```python
from build123d import *

# Parameters (mm, degrees)
SKETCH1_W           = 40
SKETCH1_H           = 40
BOSS_EXTRUDE1_DEPTH = 20
CUT_EXTRUDE1_START  = 13
SKETCH2_R           = 2.05
CUT_EXTRUDE1_DEPTH  = 34
BOSS_EXTRUDE2_DEPTH = 10
FILLET1_R           = 10
CHAMFER1_SIZE       = 1
FILLET2_R           = 3


with BuildPart() as part:
    # Sketch1 → Boss-Extrude1 (new body, symmetric)
    with BuildSketch(Plane(origin=(0, 0, 0), x_dir=(1, 0, 0), z_dir=(0, 1, 0))):
        Rectangle(SKETCH1_W, SKETCH1_H)
    extrude(amount=BOSS_EXTRUDE1_DEPTH, both=True)

    # Sketch2 → Cut-Extrude1 (cut, through all)
    with BuildSketch(Plane(origin=(0, 0, 0), x_dir=(0, 0, -1), z_dir=(1, 0, 0)).offset(CUT_EXTRUDE1_START)):
        with Locations((-7.5, 10)):
            Circle(SKETCH2_R)
        with Locations((7.5, 10)):
            Circle(SKETCH2_R)
        with Locations((-7.5, -10)):
            Circle(SKETCH2_R)
        with Locations((7.5, -10)):
            Circle(SKETCH2_R)
    cut_extrude1 = extrude(amount=-CUT_EXTRUDE1_DEPTH, mode=Mode.SUBTRACT)

    # Mirror1: Cut-Extrude1 across plane
    add(cut_extrude1.mirror(Plane(origin=(0, 0, 0), x_dir=(0, 0, 1), z_dir=(1, 0, 0))), mode=Mode.SUBTRACT)

    # Sketch3 → Boss-Extrude2 (add)
    with BuildSketch(Plane(origin=(0, 20, 0), x_dir=(1, 0, 0), z_dir=(0, 1, 0))):
        with BuildLine():
            Line((18.68, 3.6), (8.4, 3.6))
            Line((8.4, 3.6), (8.4, -3.6))
            Line((8.4, -3.6), (18.68, -3.6))
            ThreePointArc((18.68, -3.6), (19.408599647, -3.761942699), (20, -4.2172761))
            Line((20, -4.2172761), (20, 4.2172761))
            ThreePointArc((20, 4.2172761), (19.408599647, 3.761942699), (18.68, 3.6))
        make_face()
        with BuildLine():
            ThreePointArc((3.6, 18.68), (3.761942699, 19.408599647), (4.2172761, 20))
            Line((4.2172761, 20), (-4.2172761, 20))
            ThreePointArc((-4.2172761, 20), (-3.761942699, 19.408599647), (-3.6, 18.68))
            Line((-3.6, 18.68), (-3.6, 8.4))
            Line((-3.6, 8.4), (3.6, 8.4))
            Line((3.6, 8.4), (3.6, 18.68))
        make_face()
        with BuildLine():
            Line((-4.2172761, -20), (4.2172761, -20))
            ThreePointArc((4.2172761, -20), (3.761942699, -19.408599647), (3.6, -18.68))
            Line((3.6, -18.68), (3.6, -8.4))
            Line((3.6, -8.4), (-3.6, -8.4))
            Line((-3.6, -8.4), (-3.6, -18.68))
            ThreePointArc((-3.6, -18.68), (-3.761942699, -19.408599647), (-4.2172761, -20))
        make_face()
        with BuildLine():
            ThreePointArc((-18.68, 3.6), (-19.408599647, 3.761942699), (-20, 4.2172761))
            Line((-20, 4.2172761), (-20, -4.2172761))
            ThreePointArc((-20, -4.2172761), (-19.408599647, -3.761942699), (-18.68, -3.6))
            Line((-18.68, -3.6), (-8.4, -3.6))
            Line((-8.4, -3.6), (-8.4, 3.6))
            Line((-8.4, 3.6), (-18.68, 3.6))
        make_face()
    extrude(amount=BOSS_EXTRUDE2_DEPTH)

    # Fillet1
    fillet1_edges = [part.edges().sort_by_distance(p)[0] for p in [
        (0, -20, -20),
    ]]
    fillet(fillet1_edges, radius=FILLET1_R)

    # Chamfer1
    chamfer1_edges = [part.edges().sort_by_distance(p)[0] for p in [
        (-20, 10, -5.45),
        (-20, -10, 9.55),
        (-20, -10, -5.45),
        (-20, 10, 9.55),
        (20, 10, -5.45),
        (20, -10, 9.55),
        (20, -10, -5.45),
        (20, 10, 9.55),
    ]]
    chamfer(chamfer1_edges, length=CHAMFER1_SIZE)

    # Fillet2
    fillet2_edges = [part.edges().sort_by_distance(p)[0] for p in [
        (8.4, 25, -3.6),
        (8.4, 25, 3.6),
        (-8.4, 25, 3.6),
        (-8.4, 25, -3.6),
        (-3.6, 25, -8.4),
        (3.6, 25, -8.4),
        (3.6, 25, 8.4),
        (-3.6, 25, 8.4),
    ]]
    fillet(fillet2_edges, radius=FILLET2_R)


solid = part.part
```
For this review, take the finished solid that the model builds, in its own axes (mm). A direction names the side the tool comes from. Round coordinates to 2 decimals unless told otherwise and drop trailing zeros. Order: outer loops, then holes, each group sorted by start corner. A loop starts at its lowest first (then second) coordinate and runs counter-clockwise, first axis right, second up. Notation, with made-up numbers: (71, 23.25) -> (82, 23.25) arc R25 ccw to (82, 44.25) -> close; hole circle Ø8 at (89, -34). An arc over 180 degrees is marked (long way). Use a Markdown table: item, result.
Item 1: Take a section at C-C (x = 5.5). State the section outline as (y, z) points, plus the area to 3 significant figures.
Resolved:
| item | result |
|---|---|
| outline | (-20, -10) arc R10 ccw to (-10, -20) -> (20, -20) -> (20, 20) -> (-20, 20) -> close; hole circle Ø4.1 at (-10, -7.5); hole circle Ø4.1 at (-10, 7.5); hole circle Ø4.1 at (10, -7.5); hole circle Ø4.1 at (10, 7.5) |
| area | 1,530 mm² |
Item 2: Take a section at B-B (z = 7.5). State the section outline as (x, y) points.
Resolved:
| item | result |
|---|---|
| outline | (-20, -20) -> (20, -20) -> (20, -13.05) -> (19, -12.05) -> (-19, -12.05) -> (-20, -13.05) -> close; (-20, -6.95) -> (-19, -7.95) -> (19, -7.95) -> (20, -6.95) -> (20, 6.95) -> (19, 7.95) -> (-19, 7.95) -> (-20, 6.95) -> close; (-20, 13.05) -> (-19, 12.05) -> (19, 12.05) -> (20, 13.05) -> (20, 20) -> (-20, 20) -> close |
Item 3: For pin 1 (6 mm diameter, centred on x = -13.5, y = 25, fed in from -Z); pin 2 (4.5 mm diameter, centred on y = -10, z = 7.5, fed in from +X); pin 3 (6 mm diameter, centred on y = 23.5, z = 14, fed in from -X), all flat-tipped, find the tip position at first contact; note any pin that passes through.
Resolved:
| item | result |
|---|---|
| pin 1 | stops at z = -3.6 |
| pin 2 | stops at x = 19.2 |
| pin 3 | stops at x = -3.6 |
Item 4: Draft analysis for pull direction X (two halves, no side actions). For faces 5 (the cylindrical face through (3.76, 24.93, -19.4)), 6 (the flat face through (15, 25, -3.6)), 7 (the flat face through (-14, 30, 0)), state which applies: +X half, -X half, draft (parallel to the pull), parting line (faces both ways), or undercut.
Resolved:
| item | result |
|---|---|
| face 5 | +X half |
| face 6 | undercut |
| face 7 | draft |
Item 5: For line 1 along Y through (x, z) = (7.5, -7.5); line 2 along Z through (x, y) = (9, -10); line 3 along Z through (x, y) = (3, 8.5), list the stretches that pass through material, from the lowest coordinate up. Write a range as [from, to].
Resolved:
| item | result |
|---|---|
| line 1 | y = [-20, -12.05], [-7.95, 7.95], [12.05, 20] |
| line 2 | z = [-20, -9.55], [-5.45, 5.45], [9.55, 20] |
| line 3 | z = [-20, -8.9], [-6.1, 6.1], [8.9, 20] |
Item 6: Machinability: for faces 1 (the cylindrical face through (-9.3, 25.07, 2.74)), 2 (the flat face through (-8.4, 25, 0)), 3 (the flat face through (0, 25, -8.4)), 4 (the cylindrical face through (-9.26, 25.07, -2.7)), which of the approach directions +Z, -Z, +X, -X, +Y, -Y give a long, thin tool a straight path to every point of the face, cutting with its end or side? Answer none if there is none.
Resolved:
| item | result |
|---|---|
| face 1 | +Z, +Y |
| face 2 | +Z, -Z, +Y |
| face 3 | +X, -X, +Y |
| face 4 | -Z, +Y |
Item 7: Take a section at D-D (y = 23.5). State how many separate pieces and enclosed holes the cut face has, plus the area to 3 significant figures.
Resolved:
| item | result |
|---|---|
| separate pieces | 4 |
| enclosed holes | 0 |
| area | 321 mm² |
Item 8: Take a section at A-A (y = 10). State the section outline as (x, z) points.
Resolved:
| item | result |
|---|---|
| outline | (-20, -20) -> (20, -20) -> (20, -10.55) -> (19, -9.55) -> (-19, -9.55) -> (-20, -10.55) -> close; (-20, -4.45) -> (-19, -5.45) -> (19, -5.45) -> (20, -4.45) -> (20, 4.45) -> (19, 5.45) -> (-19, 5.45) -> (-20, 4.45) -> close; (-20, 10.55) -> (-19, 9.55) -> (19, 9.55) -> (20, 10.55) -> (20, 20) -> (-20, 20) -> close |
